Read the model definition and answer for the solid it produces. Units are mm, in the model's axes. A direction names the side the tool comes from. Coordinates: 2 decimals unless noted, no trailing zeros. Loops run counter-clockwise (first coordinate to the right, second up) from the corner with the lowest first, then second, coordinate; pieces in that order, holes last. Notation, with made-up numbers: (33.5, -31) -> (50.5, -31) arc R18 cw to (50.5, -1) -> close; hole circle Ø9 at (-27, -21). An arc over 180 degrees is marked (long way). Answer as a JSON object with one key per item and string values. Group by question number.
1) Flat-ended cylindrical pins translate along their axes: P1, Ø1.5, axis at x = -2.5, z = -4, coming from the +Y side; P2, Ø2, axis at x = 3.5, y = -1, coming from the -Z side; P3, Ø1.5, axis at x = 1.5, y = -1, coming from the -Z side. Find the tip coordinate at first contact, or state that the pin passes through.
2) Section B-B, the plane y = -0.25 is taken. Give the vertices of the cut face in (x, z), plus the area to 3 significant figures.
3) Determine the mould class of faces 1 (the face through (0, -2, 0)), 2 (the face through (-3, 4, 0)), 3 (the face through (0, 8, 0)) for opening direction Z: released by +Z, released by -Z, zero draft, split by the parting line, or undercut.
4) Section C-C, the plane y = 1.75 is taken. Give the vertices of the cut face in (x, z).
5) Section A-A, the plane z = 0 is taken. Give the vertices of the cut face in (x, y).
6) Consider probe 1 along Y at (x, z) = (1.5, -1.5); probe 2 along Y at (x, z) = (4, 0.25); probe 3 along Z at (x, y) = (0.5, -4.5). Determine where each line is inside the solid, lowest interval first. Write a range as [from, to].
7) Which of the six approach directions +Z, -Z, +X, -X, +Y, -Y give full straight-line access (tool end or side, diameter ignored) to faces 4 (the face through (1.233, -4.028, -2.175)), 5 (the face through (-1.08, -2.71, -4.88)), 6 (the face through (-0.1, 0, -3.3))?
from build123d import *

# Parameters (mm, degrees)
F0_R     = 5
F0_R_2   = 3
F1_DEPTH = 6
F2_DEPTH = 8
F3_SIZE  = 0.5
F5_DEPTH = 4


with BuildPart() as f1:
    # F0 (on Front) → F1 (new body)
    with BuildSketch(Plane.XZ):
        Circle(F0_R)
        Circle(F0_R_2, mode=Mode.SUBTRACT)
        Circle(F0_R_2)
    extrude(amount=F1_DEPTH)

    # F0 (on Front) → F2 (join)
    with BuildSketch(Plane.XZ):
        Circle(F0_R_2)
    extrude(amount=-F2_DEPTH)

    # F3
    f3_edges = [f1.edges().sort_by_distance(p)[0] for p in [
        (-5, -6, 0),
        (-3, 8, 0),
    ]]
    chamfer(f3_edges, length=F3_SIZE)

    # F4 (on face) → F5 (cut)
    with BuildSketch(Plane.XZ.offset(6)):
        Polygon((2.5, -1.443376), (2.5, 1.443376), (0, 2.886751), (-2.5, 1.443376), (-2.5, -1.443376), (0, -2.886751), align=None)
    extrude(amount=-F5_DEPTH, mode=Mode.SUBTRACT)


solid = f1.part
Determined:
{
 "1": {"P1": "y = 0", "P2": "z = -4.33", "P3": "z = -4.94"},
 "2": {"outline": "circle Ø10 at (0, 0)", "area": "78.5 mm²"},
 "3": {"face 1": "undercut", "face 2": "split by the parting line", "face 3": "zero draft"},
 "4": {"outline": "circle Ø6 at (0, 0)"},
 "5": {"outline": "(-5, -5.5) -> (-4.5, -6) -> (-2.5, -6) -> (-2.5, -2) -> (2.5, -2) -> (2.5, -6) -> (4.5, -6) -> (5, -5.5) -> (5, 0) -> (3, 0) -> (3, 7.5) -> (2.5, 8) -> (-2.5, 8) -> (-3, 7.5) -> (-3, 0) -> (-5, 0) -> close"},
 "6": {"probe 1": "[-2, 8]", "probe 2": "[-6, 0]", "probe 3": "[-4.97, -2.6], [2.6, 4.97]"},
 "7": {"face 4": "-Y", "face 5": "+Y, -Y", "face 6": "+Y"}
}
